Check sheet for the modelled part. Datum: model origin and axes. Units: mm. Face numbers are marked on the shaded views. Round coordinates to 2 decimals unless told otherwise and drop trailing zeros. Write each loop counter-clockwise with the first axis right and the second up, starting at its lowest first coordinate (ties: lowest second). Pieces come first, ordered by that corner, then holes.
Item 1: Release check for a two-part mould opening along X. For the marked faces 1, 2, 3 and 4 record: +X half, -X half, draft (parallel to the pull), parting line (faces both ways), or undercut.
Item 2: Cross-section at B-B on x = 2.1. Enter the section's corners in (y, z), plus the area to 3 significant figures.
Item 3: Cross-section at D-D on z = -3.8. Enter the section's corners in (x, y).
Item 4: Go/stop test with flat-tipped pins: pin 1 Ø2.5 at (x, z) = (2.5, -1.44) entering from -Y; pin 2 Ø2 at (x, y) = (2, 7) entering from -Z. Record where each tip stops, or that it passes through.
Item 5: Material ranges on line 1 (X direction, y = 17.75, z = -1.45); line 2 (X direction, y = 16.25, z = -0.7); line 3 (Z direction, x = 1.55, y = 19), recorded low to high.
Item 6: Cross-section at C-C on z = -1.55. Enter the section's corners in (x, y).
Item 7: Cross-section at A-A on y = 4.5. Enter the section's corners in (x, z).
Autodesk Inventor part; units mm, degrees
ref_plane "YZ Plane" through (0, 0, 0) normal (1, 0, 0) x (0, 1, 0)
ref_plane "XY Plane" through (0, 0, 0) normal (0, 0, 1) x (1, 0, 0)
sketch "Skizze1" plane through (0, 0, 0) normal (0, 1, 0) x (-1, 0, 0)
  line L0 (0, 0) -> (0, -2.8868)
  line L1 (0, -2.8868) -> (-2.5, -4.3301)
  line L2 (-2.5, -4.3301) -> (-5, -2.8868)
  line L3 (-5, -2.8868) -> (-5, 0)
  line L4 (-5, 0) -> (-2.5, 1.4434)
  line L5 (-2.5, 1.4434) -> (0, 0)
  dimension "d2" = 120
  dimension "d4" = 120
  dimension "d6" = 120
  dimension "d8" = 120
  dimension "d11" = 5
  dimension "d12" = 5
  dimension "d13" = 5
extrude "Extrusion1" add sketch "Skizze1" along normal blind 22
sketch "Skizze2" plane through (0, 22, 0) normal (0, 1, 0) x (1, 0, 0)
  line L0 (0, 2.8868) -> (0, 0)
  line L1 (5, 0) -> (5, 2.8868)
  line L2 (0, 0) -> (5, 2.8868) construction
  line L3 (0, 2.8868) -> (5, 0) construction
  point P0 (2.5, 1.4434)
hole "Bohrung1" at (2.5, 22, -1.4434) direction (0, -1, 0) diameter 3 end through all
thread "Gewinde1"
properties part number "abstandshalter_22mm"
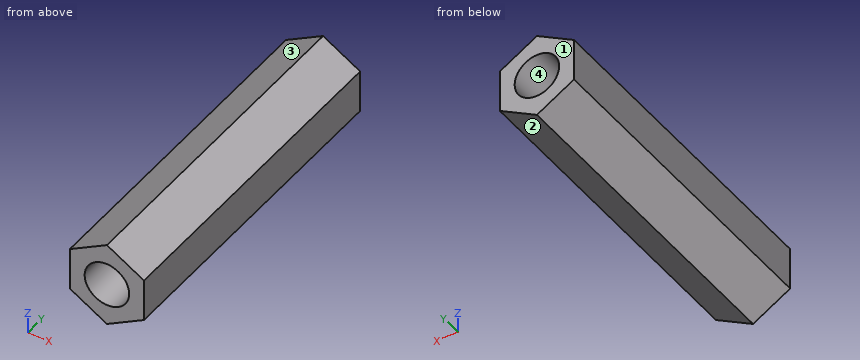
Response values:
1. face 1: draft
1. face 2: +X half
1. face 3: -X half
1. face 4: undercut
2. outline: (0, -4.1) - (22, -4.1) - (22, -2.89) - (0, -2.89) - close; (0, 0) - (22, 0) - (22, 1.21) - (0, 1.21) - close
2. area: 53.2 mm2
3. outline: (1.58, 0) - (3.42, 0) - (3.42, 22) - (1.58, 22) - close
4. pin 1: passes through
4. pin 2: stops at z = -4.33
5. line 1: x = 0 to 1, 4 to 5
5. line 2: x = 0 to 1.2, 3.8 to 5
5. line 3: z = -3.78 to -2.6, -0.28 to 0.89
6. outline: (0, 0) - (1, 0) - (1, 22) - (0, 22) - close; (4, 0) - (5, 0) - (5, 22) - (4, 22) - close
7. outline: (0, -2.89) - (2.5, -4.33) - (5, -2.89) - (5, 0) - (2.5, 1.44) - (0, 0) - close; hole circle Ø3 at (2.5, -1.44)
